from build123d import *

# Parameters (mm, degrees)
MODEL_R                 = 6
MODEL_W                 = 24
MODEL_H                 = 3
SALIENTE_EXTRUIR1_DEPTH = 3


with BuildPart() as part:
    # Model → Saliente-Extruir1 (new body)
    with BuildSketch(Plane.XY):
        Polygon((54, 89), (54, 81.9), (65.8, 81.9), (65.8, 58.7), (54, 58.7), (54, -69), (146, -69), (146, 58.7), (134.2, 58.7), (134.2, 81.9), (146, 81.9), (146, 89), align=None)
        with Locations((99.899304233, 61.529562992)):
            Circle(MODEL_R, mode=Mode.SUBTRACT)
        with Locations((100, 80.5)):
            Rectangle(MODEL_W, MODEL_H, mode=Mode.SUBTRACT)
        Polygon((85.5, 28.721585816), (85.5, 34.721585816), (90, 34.721585816), (90, 42.721585816), (85.5, 42.721585816), (85.5, 48.721585816), (74.5, 48.721585816), (74.5, 42.721585816), (70, 42.721585816), (70, 34.721585816), (74.5, 34.721585816), (74.5, 28.721585816), align=None, mode=Mode.SUBTRACT)
        Polygon((125.5, 28.721575199), (125.5, 34.721575199), (130, 34.721575199), (130, 42.721575199), (125.5, 42.721575199), (125.5, 48.721575199), (114.5, 48.721575199), (114.5, 42.721575199), (110, 42.721575199), (110, 34.721575199), (114.5, 34.721575199), (114.5, 28.721575199), align=None, mode=Mode.SUBTRACT)
    extrude(amount=SALIENTE_EXTRUIR1_DEPTH)


solid = part.part
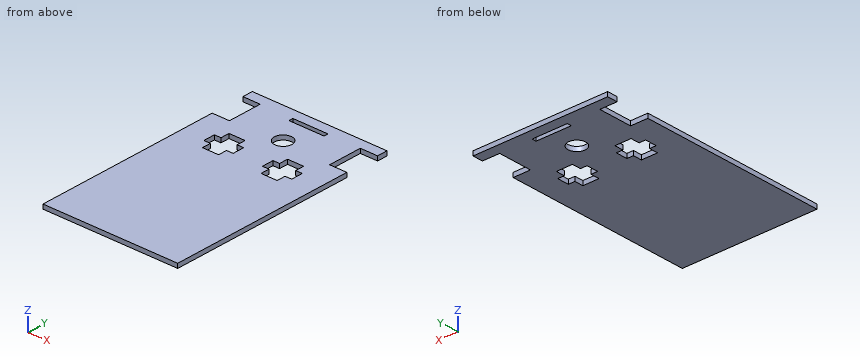
Read the model definition and answer for the solid it produces. Units are mm, in the model's axes. Round coordinates to 2 decimals unless told otherwise and drop trailing zeros. Order: outer loops, then holes, each group sorted by start corner. A loop starts at its lowest first (then second) coordinate and runs counter-clockwise, first axis right, second up.
1) The part is cut by section D-D on y = 72.5. Write down the section's boundary in (x, z), plus the area to 3 significant figures.
2) Flat-ended cylindrical pins translate along their axes: pin 1 (0.9 mm diameter, centred on y = 80, z = 2, fed in from +X); pin 2 (1.5 mm diameter, centred on y = 66, z = 1, fed in from -X); pin 3 (1 mm diameter, centred on x = 130.5, y = 2, fed in from -Z). Find the tip coordinate at first contact, or state that the pin passes through.
3) The part is cut by section A-A on x = 127.5. Write down the section's boundary in (y, z), plus the area to 3 significant figures.
4) Straight lines are drawn through the part: L1, parallel to X at y = 31.5, z = 2.45; L2, parallel to Y at x = 71, z = 2.8; L3, parallel to Y at x = 140.5, z = 1.05. For each, find the intervals that lie inside material, in ascending order.
5) The part is cut by section B-B on y = 37.5. Write down the section's boundary in (x, z).
6) The part is cut by section C-C on x = 83.5. Write down the section's boundary in (y, z), plus the area to 3 significant figures.
Resolved:
1. outline: (65.8, 0) - (134.2, 0) - (134.2, 3) - (65.8, 3) - close
1. area: 205 mm2
2. pin 1: stops at x = 134.2
2. pin 2: stops at x = 65.8
2. pin 3: stops at z = 0
3. outline: (-69, 0) - (34.72, 0) - (34.72, 3) - (-69, 3) - close; (42.72, 0) - (89, 0) - (89, 3) - (42.72, 3) - close
3. area: 450 mm2
4. L1: x = 54 to 74.5, 85.5 to 114.5, 125.5 to 146
4. L2: y = -69 to 34.72, 42.72 to 89
4. L3: y = -69 to 58.7, 81.9 to 89
5. outline: (54, 0) - (70, 0) - (70, 3) - (54, 3) - close; (90, 0) - (110, 0) - (110, 3) - (90, 3) - close; (130, 0) - (146, 0) - (146, 3) - (130, 3) - close
6. outline: (-69, 0) - (28.72, 0) - (28.72, 3) - (-69, 3) - close; (48.72, 0) - (89, 0) - (89, 3) - (48.72, 3) - close
6. area: 414 mm2
